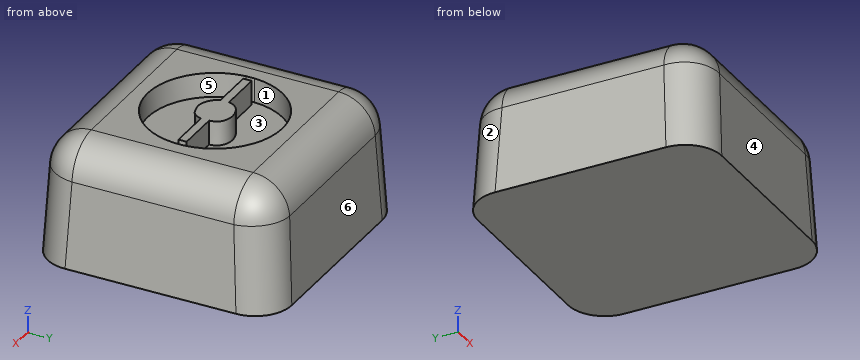
from build123d import *

# Parameters (mm, degrees)
F0_W     = 20
F0_H     = 20
F1_DEPTH = 10
F1_TAPER = 3
F2_R     = 3
F4_DEPTH = 2


with BuildPart() as f1:
    # F0 (on Top) → F1 (new body)
    with BuildSketch(Plane.XY):
        Rectangle(F0_W, F0_H)
    extrude(amount=F1_DEPTH, taper=F1_TAPER)

    # F2
    f2_edges = [f1.edges().sort_by_distance(p)[0] for p in [
        (0, 9.475922, 10),
        (9.737961, 9.737961, 5),
        (9.475922, 0, 10),
        (9.737961, -9.737961, 5),
        (0, -9.475922, 10),
        (-9.475922, 0, 10),
        (-9.737961, -9.737961, 5),
        (-9.737961, 9.737961, 5),
    ]]
    fillet(f2_edges, radius=F2_R)

    # F3 (on face) → F4 (cut)
    with BuildSketch(Plane.XY.offset(10)):
        with BuildLine():
            ThreePointArc((5.5115809634, 0.2857532818), (0.0129202811, 5.5189684471), (-5.5101826217, 0.3115559812))
            Line((-5.5101826217, 0.3115559812), (-5.0968159921, 0.3115559812))
            Line((-5.0968159921, 0.3115559812), (-1.5841760834, 0.3115559812))
            add(Edge.make_bspline(
                [(-1.5841760834, 0.3115559812), (-1.5146037038, 0.5837301371), (-1.2273483423, 1.2298845271), (0.2804225775, 1.6685983953), (1.3624047254, 1.0479713111), (1.4321026561, 0.5130518001), (1.4605487231, 0.2857532818)],
                knots=[0, 0, 0, 0, 0.0939716444, 0.212909057, 0.3170188857, 0.399881643, 0.399881643, 0.399881643, 0.399881643], degree=3))
            Line((1.4605487231, 0.2857532818), (4.9382173456, 0.2857532818))
            Line((4.9382173456, 0.2857532818), (5.5115809634, 0.2857532818))
        make_face()
        with BuildLine():
            Line((-5.0968159921, -0.3829301172), (-5.5056828986, -0.3829301172))
            ThreePointArc((-5.5056828986, -0.3829301172), (0, -5.5189835707), (5.5056828986, -0.3829301172))
            Line((5.5056828986, -0.3829301172), (4.9382173456, -0.3829301172))
            Line((4.9382173456, -0.3829301172), (1.4605487231, -0.3829301172))
            add(Edge.make_bspline(
                [(1.4605487231, -0.3829301172), (1.400668735, -0.6466191855), (1.09179653, -1.2105707709), (0.3230563372, -1.3669788929), (-0.3039180378, -1.4893536378), (-1.0857394106, -1.1379114959), (-1.4961255451, -0.6391379868), (-1.5841760834, -0.3829301172)],
                knots=[0.480759332, 0.480759332, 0.480759332, 0.480759332, 0.5717887242, 0.6570378834, 0.7350044671, 0.8245681269, 0.917576654, 0.917576654, 0.917576654, 0.917576654], degree=3))
            Line((-1.5841760834, -0.3829301172), (-5.0968159921, -0.3829301172))
        make_face()
        Polygon((-5.5101826217, 0.3115559812), (-5.5056828986, -0.3829301172), (-5.0968159921, -0.3829301172), (-5.0968159921, 0.3115559812), align=None)
        Polygon((4.9382173456, -0.3829301172), (5.5056828986, -0.3829301172), (5.5115809634, 0.2857532818), (4.9382173456, 0.2857532818), align=None)
    extrude(amount=-F4_DEPTH, mode=Mode.SUBTRACT)


solid = f1.part
Geometry check sheet. Reference: the model listing, model coordinates, mm. Face numbers are marked on the shaded views. A direction names the side the tool comes from. Give positions to 0.01 mm unless a question says otherwise; leave off trailing zeros. Loops run counter-clockwise (first coordinate to the right, second up) from the corner with the lowest first, then second, coordinate; pieces in that order, holes last.
(1) Set-up check for the marked faces 1 and 2: record each of +Z, -Z, +X, -X, +Y, -Y from which the full face is reachable in a straight line by a thin tool's end or side.
From the geometry:
face 1: +Z
face 2: +Z, -X, +Y
(2) Depth check by flat-ended pin: pin 1 Ø1 at (x, z) = (5, 4) entering from -Y; pin 2 Ø4 at (y, z) = (-7.5, 8.5) entering from +X; pin 3 Ø0.6 at (x, z) = (3.5, 9.5) entering from +Y. Enter the tip coordinate at first touch or a pass-through.
From the geometry:
pin 1: stops at y = -9.82
pin 2: stops at x = 9.65
pin 3: stops at y = 8.67
(3) Section check C-C on z = 9. Count the separate pieces of the cut face and the enclosed holes in it, then the cut area to 3 significant figures.
From the geometry:
separate pieces: 2
enclosed holes: 1
area: 226 mm2
(4) Section check D-D on z = 7.75. Record the cut outline in (x, y), then the cut area to 3 significant figures.
From the geometry:
outline: (-9.53, -6.63) arc R2.9 ccw to (-6.63, -9.53) - (6.63, -9.53) arc R2.9 ccw to (9.53, -6.63) - (9.53, 6.63) arc R2.9 ccw to (6.63, 9.53) - (-6.63, 9.53) arc R2.9 ccw to (-9.53, 6.63) - close
area: 356 mm2
(5) Release check for a two-part mould opening along Y. For the marked faces 3, 4, 5 and 6 record: released by +Y, released by -Y, zero draft, split by the parting line, or undercut.
From the geometry:
face 3: undercut
face 4: released by -Y
face 5: undercut
face 6: released by +Y
(6) Thickness scan on L1, parallel to Y at x = 4.75, z = 8.5; L2, parallel to X at y = 2.75, z = 8.75; L3, parallel to Z at x = -3.75, y = 1.75. Record the ranges inside material, lowest first.
From the geometry:
L1: y = -9.23 to -2.81, -0.38 to 0.29, 2.81 to 9.23
L2: x = -9.07 to -4.79, 4.79 to 9.07
L3: z = 0 to 8
(7) Section check B-B on y = -2.25. Record the cut outline in (x, z), then the cut area to 3 significant figures.
From the geometry:
outline: (-10, 0) - (10, 0) - (9.62, 7.16) arc R3 ccw to (6.63, 10) - (5.04, 10) - (5.04, 8) - (-5.04, 8) - (-5.04, 10) - (-6.63, 10) arc R3 ccw to (-9.62, 7.16) - close
area: 171 mm2
(8) Section check A-A on x = 6.25. Record the cut outline in (y, z).
From the geometry:
outline: (-10, 0) - (10, 0) - (9.62, 7.16) arc R3 ccw to (6.63, 10) - (-6.63, 10) arc R3 ccw to (-9.62, 7.16) - close
